The listing builds one solid part. Answer for the finished solid, in the listing's coordinates (mm). Coordinates: 2 decimals unless noted, no trailing zeros. Loops run counter-clockwise (first coordinate to the right, second up) from the corner with the lowest first, then second, coordinate; pieces in that order, holes last. Notation, with made-up numbers: M 17.5,53 L 66.5,53 A11 ccw 66.5,72 Z; hole C -39.75,-23 d9. An arc over 180 degrees is marked long. Answer as a JSON object with one key per item and string values. Group by question number.
1. Straight lines are drawn through the part: L1, parallel to Z at x = 0, y = 0.85 (3 decimals); L2, parallel to X at y = 2.6, z = 41.5; L3, parallel to Z at x = -43, y = 2.15. For each, find the intervals that lie inside material, in ascending order.
2. Determine the mould class of faces 1 (the face through (75.71, 1.5, -23.84)), 2 (the face through (-2.67, 1.5, 66.62)), 3 (the face through (-47.4, 0, -47.4)) for opening direction Z: released by +Z, released by -Z, zero draft, split by the parting line, or undercut.
3. A cutting plane is placed at B-B on y = 1.75. State how many separate pieces and enclosed holes the cut face has, and give its area (3 significant figures).
4. A cutting plane is placed at C-C on x = -48. Give the vertices of the cut face in (y, z).
5. A cutting plane is placed at A-A on x = 17.5. Give the vertices of the cut face in (y, z), and give its area (3 significant figures).
from build123d import *

# Parameters (mm, degrees)
SKETCH2_R           = 79.375
SKETCH2_R_2         = 66.675
SKETCH2_R_3         = 1.4224
BOSS_EXTRUDE1_DEPTH = 3.048
CUT_EXTRUDE2_DEPTH  = 4.048


with BuildPart() as part:
    # Sketch2 → Boss-Extrude1 (new body)
    with BuildSketch(Plane(origin=(0, 0, 0), x_dir=(1, 0, 0), z_dir=(0, 1, 0))):
        Circle(SKETCH2_R)
        Circle(SKETCH2_R_2, mode=Mode.SUBTRACT)
        with Locations((0, 73.025)):
            Circle(SKETCH2_R_3, mode=Mode.SUBTRACT)
        with Locations((27.945457648, 67.466302862)):
            Circle(SKETCH2_R_3, mode=Mode.SUBTRACT)
        with Locations((51.636472696, 51.636472696)):
            Circle(SKETCH2_R_3, mode=Mode.SUBTRACT)
        with Locations((67.466302862, 27.945457648)):
            Circle(SKETCH2_R_3, mode=Mode.SUBTRACT)
        with Locations((73.025, 0)):
            Circle(SKETCH2_R_3, mode=Mode.SUBTRACT)
        with Locations((67.466302862, -27.945457648)):
            Circle(SKETCH2_R_3, mode=Mode.SUBTRACT)
        with Locations((51.636472696, -51.636472696)):
            Circle(SKETCH2_R_3, mode=Mode.SUBTRACT)
        with Locations((27.945457648, -67.466302862)):
            Circle(SKETCH2_R_3, mode=Mode.SUBTRACT)
        with Locations((0, -73.025)):
            Circle(SKETCH2_R_3, mode=Mode.SUBTRACT)
        with Locations((-27.945457648, -67.466302862)):
            Circle(SKETCH2_R_3, mode=Mode.SUBTRACT)
        with Locations((-51.636472696, -51.636472696)):
            Circle(SKETCH2_R_3, mode=Mode.SUBTRACT)
        with Locations((-67.466302862, -27.945457648)):
            Circle(SKETCH2_R_3, mode=Mode.SUBTRACT)
        with Locations((-73.025, 0)):
            Circle(SKETCH2_R_3, mode=Mode.SUBTRACT)
        with Locations((-67.466302862, 27.945457648)):
            Circle(SKETCH2_R_3, mode=Mode.SUBTRACT)
        with Locations((-51.636472696, 51.636472696)):
            Circle(SKETCH2_R_3, mode=Mode.SUBTRACT)
        with Locations((-27.945457648, 67.466302862)):
            Circle(SKETCH2_R_3, mode=Mode.SUBTRACT)
    extrude(amount=BOSS_EXTRUDE1_DEPTH)

    # Sketch5 → Cut-Extrude2 (cut, through all)
    with BuildSketch(Plane(origin=(0, 0, 0), x_dir=(-1, 0, 0), z_dir=(0, -1, 0))):
        with BuildLine():
            Line((20.972211437, 63.290773202), (20.941758021, 67.713419083))
            Line((20.941758021, 67.713419083), (-21.068846043, 67.42414284))
            Line((-21.068846043, 67.42414284), (-21.040229048, 63.268194115))
            ThreePointArc((-21.040229048, 63.268194115), (-0.03583368, 66.674990371), (20.972211437, 63.290773202))
        make_face()
    extrude(amount=-CUT_EXTRUDE2_DEPTH, mode=Mode.SUBTRACT)


solid = part.part
From the geometry:
{
 "1": {"L1": "z = -79.375 to -74.447, -71.603 to -67.569, 66.675 to 71.603, 74.447 to 79.375", "L2": "x = -67.66 to -52.19, 52.19 to 67.66", "L3": "z = -66.72 to -50.96, 50.96 to 66.72"},
 "2": {"face 1": "split by the parting line", "face 2": "undercut", "face 3": "zero draft"},
 "3": {"separate pieces": "1", "enclosed holes": "17", "area": "5,640 mm²"},
 "4": {"outline": "M 0,-63.22 L 3.05,-63.22 L 3.05,-46.28 L 0,-46.28 Z; M 0,46.28 L 3.05,46.28 L 3.05,63.22 L 0,63.22 Z"},
 "5": {"outline": "M 0,-77.42 L 3.05,-77.42 L 3.05,-67.45 L 0,-67.45 Z; M 0,64.34 L 3.05,64.34 L 3.05,77.42 L 0,77.42 Z", "area": "70.3 mm²"}
}
